from build123d import *

# Parameters (mm, degrees)
F0_W           = 101.6
F0_H           = 152.4
F1_DEPTH       = 12.7
F2_D           = 6.35
F2_CBORE_D     = 9.525
F2_CBORE_DEPTH = 6.35
F3_R           = 4.7498


with BuildPart() as f1:
    # F0 (on Right) → F1 (new body)
    with BuildSketch(Plane.YZ):
        Rectangle(F0_W, F0_H)
    extrude(amount=-F1_DEPTH)

    # F2 (through all)
    with Locations(Plane.YZ):
        with Locations((-41.275, -69.85), (41.275, -69.85), (-41.275, 63.5), (41.275, 63.5)):
            CounterBoreHole(F2_D / 2, F2_CBORE_D / 2, F2_CBORE_DEPTH)

    # F3
    f3_edges = [f1.edges().sort_by_distance(p)[0] for p in [
        (0, 0, 76.2),
        (0, -50.8, 0),
        (0, 50.8, 0),
        (-6.35, -50.8, 76.2),
        (-6.35, 50.8, 76.2),
    ]]
    fillet(f3_edges, radius=F3_R)


solid = f1.part
Model file for the job. Use its own axes, mm. A direction names the side the tool comes from. Round coordinates to 2 decimals unless told otherwise and drop trailing zeros.
1. Drop flat-ended pins along their axis: P1, Ø5, axis at y = 39.5, z = -70.5, coming from the +X side; P2, Ø1.5, axis at x = -3.5, z = 16.5, coming from the -Y side. Give the stop position or say it passes through.
Check values:
P1: stops at x = -6.35
P2: stops at y = -50.77
2. Wall check: probe 1 along Z at (x, y) = (-5.25, 39.5); probe 2 along Z at (x, y) = (-3, 39); probe 3 along Y at (x, z) = (-3.25, 67). Give the ranges that are in metal, low to high.
Check values:
probe 1: z = -76.2 to -74.27, -65.43 to 59.08, 67.92 to 76.2
probe 2: z = -76.2 to -74.03, -65.67 to 59.32, 67.68 to 75.87
probe 3: y = -50.56 to -44.5, -38.05 to 38.05, 44.5 to 50.56
3. Mould opens along Y. For faces 3 (the cylindrical face through (-9.57, 41.96, -72.95)), 4 (the cylindrical face through (-8.781, -49.446, 74.772)), 5 (the cylindrical face through (-1.428, 0.645, 74.846)), 6 (the cylindrical face through (-1.354, 49.372, -1.341)) say: +Y half, -Y half, draft (parallel to the pull), parting line (faces both ways), or undercut.
Check values:
face 3: undercut
face 4: -Y half
face 5: draft
face 6: +Y half
4. Tool access for faces 1 (the cylindrical face through (-3.131, 40.655, 68.222)), 2 (the cylindrical face through (-8.781, 49.372, 74.846)): list every direction of +Z, -Z, +X, -X, +Y, -Y with a clear straight run to the whole face (end or side of a thin tool).
Check values:
face 1: +X
face 2: +Z, +X, -X, +Y
5. Band-saw the part on A-A, the plane z = -69.85. Count the separate pieces of the cut face and the enclosed holes in it, and give its area (3 significant figures).
Check values:
separate pieces: 3
enclosed holes: 0
area: 1,080 mm2
